The figure shows three views and two pictorial views of one solid part (mm, origin at its lowest corner). Answer the questions. Coordinates: 2 decimals unless noted, no trailing zeros. Order: outer loops, then holes, each group sorted by start corner. A loop starts at its lowest first (then second) coordinate and runs counter-clockwise, first axis right, second up. Notation, with made-up numbers: (81.5, 41.25) -> (127.5, 41.25) arc R17 ccw to (127.5, 74.25) -> close; hole circle Ø10 at (7, -12). An arc over 180 degrees is marked (long way). Write item = value, one per line. Start each with the question number.
Q1. The part is cut by section B-B, the plane z = 12.7. Determine the outline of the cut face in (x, y), plus the area to 3 significant figures.
Q2. The part is cut by section C-C, the plane y = 37. Determine the outline of the cut face in (x, z).
Q3. Flat-ended cylindrical pins translate along their axes: pin 1 (4 mm diameter, centred on x = 8.5, z = 10, fed in from -Y); pin 2 (1.5 mm diameter, centred on x = 20, y = 36, fed in from +Z); pin 3 (3 mm diameter, centred on y = 46, z = 16.5, fed in from +X); pin 4 (3 mm diameter, centred on x = 14.5, z = 9, fed in from -Y). Find the tip coordinate at first contact, or state that the pin passes through.
Q4. Straight lines are drawn through the part: L1, parallel to Z at x = 12.7, y = 73; L2, parallel to Y at x = 4.5, z = 19; L3, parallel to X at y = 103, z = 8.5. For each, find the intervals that lie inside material, in ascending order. Write a range as from..to.
Q5. For a pull along Z with two mould halves and no side action, classify the marked faces 1 and 2 as +Z half, -Z half, draft (parallel to the pull), parting line (faces both ways), or undercut.
Q6. The part is cut by section A-A, the plane x = 12.7. Determine the outline of the cut face in (y, z).
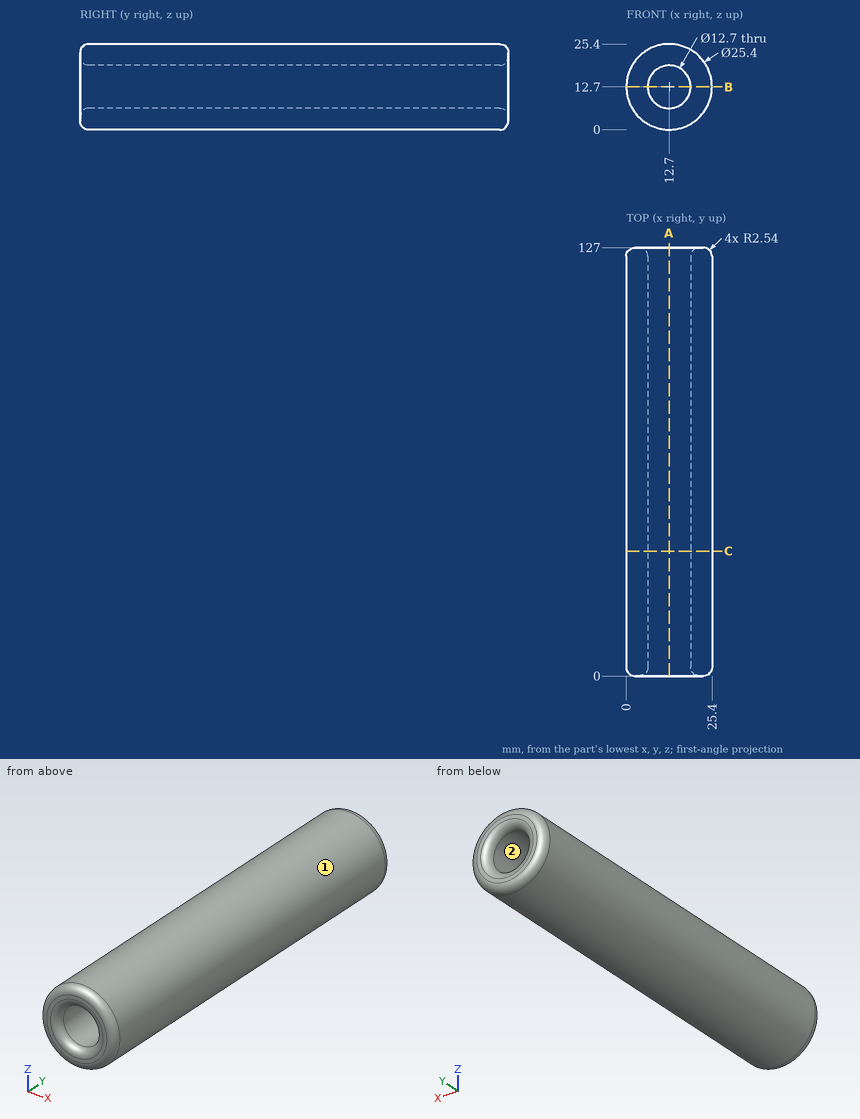
Model answer:
q1.outline = (0, 2.54) arc R2.54 ccw to (2.54, 0) -> (3.81, 0) arc R2.54 ccw to (6.35, 2.54) -> (6.35, 124.46) arc R2.54 ccw to (3.81, 127) -> (2.54, 127) arc R2.54 ccw to (0, 124.46) -> close; (19.05, 2.54) arc R2.54 ccw to (21.59, 0) -> (22.86, 0) arc R2.54 ccw to (25.4, 2.54) -> (25.4, 124.46) arc R2.54 ccw to (22.86, 127) -> (21.59, 127) arc R2.54 ccw to (19.05, 124.46) -> close
q1.area = 1,600 mm2
q2.outline = circle Ø25.4 at (12.7, 12.7); hole circle Ø12.7 at (12.7, 12.7)
q3.pin_1 = 0.85
q3.pin_2 = 23.58
q3.pin_3 = 25.19
q3.pin_4 = through
q4.L1 = 0..6.35, 19.05..25.4
q4.L2 = 0.01..126.99
q4.L3 = 0.71..7.94, 17.46..24.69
q5.face_1 = parting line
q5.face_2 = undercut
q6.outline = (0, 2.54) arc R2.54 ccw to (2.54, 0) -> (124.46, 0) arc R2.54 ccw to (127, 2.54) -> (127, 3.81) arc R2.54 ccw to (124.46, 6.35) -> (2.54, 6.35) arc R2.54 ccw to (0, 3.81) -> close; (0, 21.59) arc R2.54 ccw to (2.54, 19.05) -> (124.46, 19.05) arc R2.54 ccw to (127, 21.59) -> (127, 22.86) arc R2.54 ccw to (124.46, 25.4) -> (2.54, 25.4) arc R2.54 ccw to (0, 22.86) -> close
